Drawing for the job (mm, zero at the part's lowest x, y, z). A direction names the side the tool comes from. Round coordinates to 2 decimals unless told otherwise and drop trailing zeros. Order: outer loops, then holes, each group sorted by start corner. A loop starts at its lowest first (then second) coordinate and runs counter-clockwise, first axis right, second up. Notation, with made-up numbers: (82, -14.5) - (110, -14.5) arc R35 ccw to (110, 21.5) - close; hole circle Ø11 at (3, 88). An arc over 180 degrees is marked (long way). One line per question, with ' | ' between items. Start each with the question number.
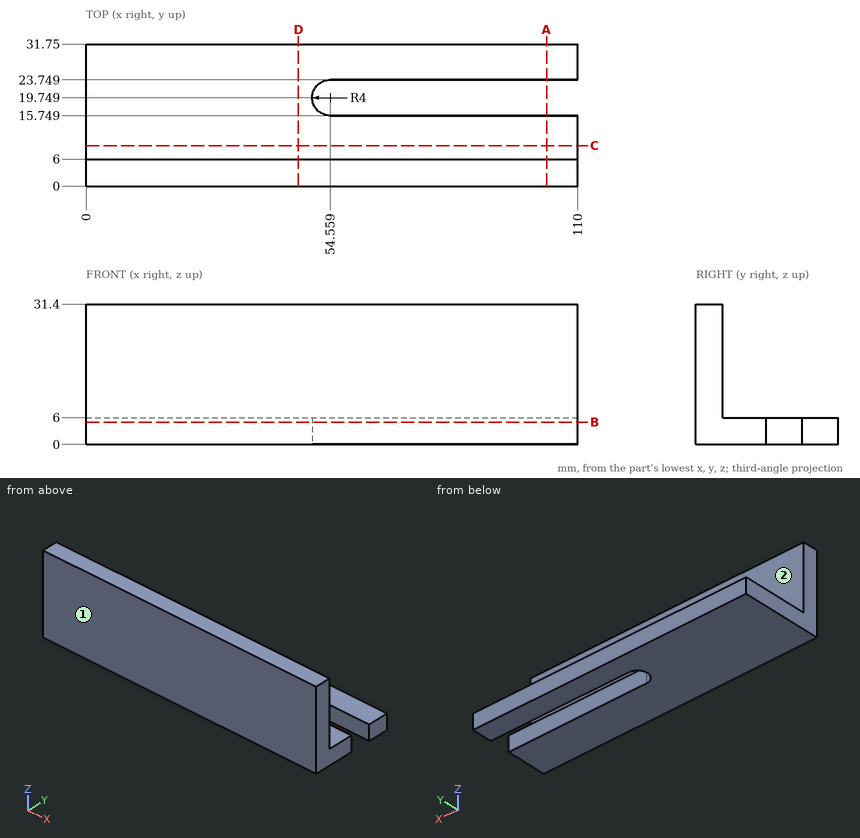
Item 1: Pin check, flat tips, straight feed: pin 1 (12 mm diameter, centred on x = 81.5, z = 27.5, fed in from +Y); pin 2 (1.5 mm diameter, centred on x = 27, y = 23, fed in from +Z); pin 3 (10 mm diameter, centred on y = 21, z = 14, fed in from -X). Stop position of each tip, or through.
Item 2: Slice it at C-C (y = 9). Write the cut outline in (x, z).
Item 3: Slice it at D-D (x = 47.5). Write the cut outline in (y, z), plus the area to 3 significant figures.
Item 4: 3-axis set-ups, long thin cutter, end or side, ignore diameter. For the marked faces 1 and 2: which of +Z, -Z, +X, -X, +Y, -Y reach the whole face in a straight line?
Item 5: Wall check: line 1 along Y through (x, z) = (71, 5); line 2 along Z through (x, y) = (80, 29). Give the ranges that are in metal, low to high. Write a range as [from, to].
Item 6: Slice it at B-B (z = 5). Write the cut outline in (x, y).
Item 7: Slice it at A-A (x = 103). Write the cut outline in (y, z), plus the area to 3 significant figures.
A:
1) pin 1: y = 6 | pin 2: z = 6 | pin 3: through
2) outline: (0, 0) - (110, 0) - (110, 6) - (0, 6) - close
3) outline: (0, 0) - (31.75, 0) - (31.75, 6) - (6, 6) - (6, 31.4) - (0, 31.4) - close | area: 343 mm^2
4) face 1: +Z, -Z, +X, -X, -Y | face 2: +Z, +X, -X, +Y
5) line 1: [0, 15.75], [23.75, 31.75] | line 2: [0, 6]
6) outline: (0, 0) - (110, 0) - (110, 15.75) - (54.56, 15.75) arc R4 cw to (54.56, 23.75) - (110, 23.75) - (110, 31.75) - (0, 31.75) - close
7) outline: (0, 0) - (15.75, 0) - (15.75, 6) - (6, 6) - (6, 31.4) - (0, 31.4) - close; (23.75, 0) - (31.75, 0) - (31.75, 6) - (23.75, 6) - close | area: 295 mm^2
